from build123d import *

# Parameters (mm, degrees)
SKETCH1_R           = 30
BOSS_EXTRUDE1_DEPTH = 10
CUT_EXTRUDE1_REACH  = 12
SKETCH2_R           = 1.25
CUT_EXTRUDE4_DEPTH  = 10
CIRPATTERN2_COUNT   = 7


with BuildPart() as part:
    # Sketch1 → Boss-Extrude1 (new body)
    with BuildSketch(Plane(origin=(0, 0, 0), x_dir=(1, 0, 0), z_dir=(0, 1, 0))):
        Circle(SKETCH1_R)
    extrude(amount=BOSS_EXTRUDE1_DEPTH)

    # Sketch2 → Cut-Extrude1 (cut, up to next)
    with BuildSketch(Plane(origin=(0, 10, 0), x_dir=(1, 0, 0), z_dir=(0, 1, 0)), mode=Mode.PRIVATE) as cut_extrude1_sk1:
        with Locations((-7.753929223, 5.488768678)):
            Circle(SKETCH2_R)
    cut_extrude1_tool1 = extrude(cut_extrude1_sk1.sketch, amount=-CUT_EXTRUDE1_REACH, mode=Mode.PRIVATE) & part.part
    add(cut_extrude1_tool1.solids().sort_by_distance((-7.753929, 10, -5.488769))[0], mode=Mode.SUBTRACT)
    # Sketch2 → Cut-Extrude1 (cut, up to next)
    with BuildSketch(Plane(origin=(0, 10, 0), x_dir=(1, 0, 0), z_dir=(0, 1, 0)), mode=Mode.PRIVATE) as cut_extrude1_sk2:
        with Locations((0.876448499, 9.459484025)):
            Circle(SKETCH2_R)
    cut_extrude1_tool2 = extrude(cut_extrude1_sk2.sketch, amount=-CUT_EXTRUDE1_REACH, mode=Mode.PRIVATE) & part.part
    add(cut_extrude1_tool2.solids().sort_by_distance((0.876448, 10, -9.459484))[0], mode=Mode.SUBTRACT)
    # Sketch2 → Cut-Extrude1 (cut, up to next)
    with BuildSketch(Plane(origin=(0, 10, 0), x_dir=(1, 0, 0), z_dir=(0, 1, 0)), mode=Mode.PRIVATE) as cut_extrude1_sk3:
        with Locations((8.630377722, 3.970715347)):
            Circle(SKETCH2_R)
    cut_extrude1_tool3 = extrude(cut_extrude1_sk3.sketch, amount=-CUT_EXTRUDE1_REACH, mode=Mode.PRIVATE) & part.part
    add(cut_extrude1_tool3.solids().sort_by_distance((8.630378, 10, -3.970715))[0], mode=Mode.SUBTRACT)
    # Sketch2 → Cut-Extrude1 (cut, up to next)
    with BuildSketch(Plane(origin=(0, 10, 0), x_dir=(1, 0, 0), z_dir=(0, 1, 0)), mode=Mode.PRIVATE) as cut_extrude1_sk4:
        with Locations((7.753929223, -5.488768678)):
            Circle(SKETCH2_R)
    cut_extrude1_tool4 = extrude(cut_extrude1_sk4.sketch, amount=-CUT_EXTRUDE1_REACH, mode=Mode.PRIVATE) & part.part
    add(cut_extrude1_tool4.solids().sort_by_distance((7.753929, 10, 5.488769))[0], mode=Mode.SUBTRACT)
    # Sketch2 → Cut-Extrude1 (cut, up to next)
    with BuildSketch(Plane(origin=(0, 10, 0), x_dir=(1, 0, 0), z_dir=(0, 1, 0)), mode=Mode.PRIVATE) as cut_extrude1_sk5:
        with Locations((-0.876448499, -9.459484025)):
            Circle(SKETCH2_R)
    cut_extrude1_tool5 = extrude(cut_extrude1_sk5.sketch, amount=-CUT_EXTRUDE1_REACH, mode=Mode.PRIVATE) & part.part
    add(cut_extrude1_tool5.solids().sort_by_distance((-0.876448, 10, 9.459484))[0], mode=Mode.SUBTRACT)
    # Sketch2 → Cut-Extrude1 (cut, up to next)
    with BuildSketch(Plane(origin=(0, 10, 0), x_dir=(1, 0, 0), z_dir=(0, 1, 0)), mode=Mode.PRIVATE) as cut_extrude1_sk6:
        with Locations((-8.630377722, -3.970715347)):
            Circle(SKETCH2_R)
    cut_extrude1_tool6 = extrude(cut_extrude1_sk6.sketch, amount=-CUT_EXTRUDE1_REACH, mode=Mode.PRIVATE) & part.part
    add(cut_extrude1_tool6.solids().sort_by_distance((-8.630378, 10, 3.970715))[0], mode=Mode.SUBTRACT)

    # Sketch6 → Cut-Extrude4 (cut)
    with BuildSketch(Plane(origin=(0, 10, 0), x_dir=(1, 0, 0), z_dir=(0, 1, 0))):
        with BuildLine():
            ThreePointArc((24.68695866, -2.287317978), (16.889428305, -10.428386728), (5.851580512, -12.71845138))
            ThreePointArc((5.851580512, -12.71845138), (15.949007833, -13.13834176), (25.324062707, -9.36439256))
            ThreePointArc((25.324062707, -9.36439256), (26.329710343, -5.978825407), (26.884849336, -2.490958893))
            Line((26.884849336, -2.490958893), (24.68695866, -2.287317978))
        make_face()
        with BuildLine():
            ThreePointArc((26.613477911, 4.552229506), (25.97279828, 1.041593529), (24.68695866, -2.287317978))
            Line((24.68695866, -2.287317978), (26.884849336, -2.490958893))
            ThreePointArc((26.884849336, -2.490958893), (26.979981102, 1.039528618), (26.613477911, 4.552229506))
        make_face()
    cut_extrude4 = extrude(amount=-CUT_EXTRUDE4_DEPTH, mode=Mode.SUBTRACT)

    # CirPattern2: Cut-Extrude4 ×7 about axis
    cirpattern2_axis = Axis((-0.506628383, 0, -0.191712569), (0, 1, 0))
    for i in range(1, CIRPATTERN2_COUNT):
        add(cut_extrude4.rotate(cirpattern2_axis, i * 360 / CIRPATTERN2_COUNT), mode=Mode.SUBTRACT)


solid = part.part
Could you check a few things on this model? Use its own coordinates, in mm. Give positions to 0.01 mm unless a question says otherwise; leave off trailing zeros. Write each loop counter-clockwise with the first axis right and the second up, starting at its lowest first coordinate (ties: lowest second). Pieces come first, ordered by that corner, then holes. Notation, with made-up numbers: (70, 12) -> (128, 12) arc R26 ccw to (128, 31) -> close; hole circle Ø9 at (34, 3). An arc over 180 degrees is marked (long way). Answer as a JSON object with one key per item and string values.
Q1. Suppose I cut it at A-A on z = 0. Write out the boundary of the cut face in (x, y), then the cut area to 3 significant figures.
Taken from the geometry:
{"outline": "(-30, 0) -> (-26.32, 0) -> (-26.32, 10) -> (-30, 10) -> close; (-22.14, 0) -> (15.85, 0) -> (15.85, 10) -> (-22.14, 10) -> close; (16.75, 0) -> (25.65, 0) -> (25.65, 10) -> (16.75, 10) -> close; (27, 0) -> (30, 0) -> (30, 10) -> (27, 10) -> close", "area": "536 mm²"}
Q2. Will these pins go through, and if not, where does the flat tip stop? pin 1 Ø3 at (y, z) = (6, -19) entering from +X; pin 2 Ø2 at (x, z) = (-7.75, -5.49) entering from +Y; pin 3 Ø5 at (x, y) = (0, 5) entering from -Z; pin 4 Ø1 at (y, z) = (9, -17.5) entering from +X.
Taken from the geometry:
{"pin 1": "stops at x = 24.37", "pin 2": "passes through", "pin 3": "stops at z = -30", "pin 4": "stops at x = 24.72"}
Q3. Please list where these lines run through material, in increasing order: L1, parallel to X at y = 6, z = 5; L2, parallel to Z at x = -3, y = 6; L3, parallel to X at y = 1, z = 18.
Taken from the geometry:
{"L1": "x = -29.58 to -27.55, -23.91 to -15.38, -15.02 to -9.34, -7.92 to 6.6, 8.9 to 23.04, 26.53 to 29.58", "L2": "z = -29.85 to -27.61, -25.12 to -16.35, -15.8 to 16.96, 18.6 to 26.98, 27.17 to 29.85", "L3": "x = -24 to -16.89, -13.28 to -3.49, -1.65 to 24"}
Q4. Suppose I cut it at C-C on y = 4.5. Count the separate pieces of the cut face and the enclosed holes in it, then the cut area to 3 significant figures.
Taken from the geometry:
{"separate pieces": "1", "enclosed holes": "13", "area": "2,340 mm²"}
Q5. Suppose I cut it at B-B on x = -18. Write out the boundary of the cut face in (y, z), then the cut area to 3 significant figures.
Taken from the geometry:
{"outline": "(0, -24) -> (10, -24) -> (10, -20.19) -> (0, -20.19) -> close; (0, -15.79) -> (10, -15.79) -> (10, -6.94) -> (0, -6.94) -> close; (0, -5.35) -> (10, -5.35) -> (10, 24) -> (0, 24) -> close", "area": "420 mm²"}
